Geometry check sheet. Reference: the model listing, model coordinates, mm. A direction names the side the tool comes from. Round coordinates to 2 decimals unless told otherwise and drop trailing zeros. Order: outer loops, then holes, each group sorted by start corner. A loop starts at its lowest first (then second) coordinate and runs counter-clockwise, first axis right, second up. Notation, with made-up numbers: M 26.25,47.5 L 48.25,47.5 A26 cw 48.25,86.5 Z; hole C 65.25,-21 d10. An arc over 180 degrees is marked long. Return JSON: item names as keys, results as strings. Group by question number.
```python
from build123d import *

# Parameters (mm, degrees)
SKETCH1_R           = 11.5
BOSS_EXTRUDE1_DEPTH = 5.3
BOSS_EXTRUDE2_START = 1
SKETCH2_R           = 11.5
BOSS_EXTRUDE2_DEPTH = 1
BOSS_EXTRUDE3_DEPTH = 6.3
FILLET1_R           = 5
CHAMFER1_SIZE       = 1
CUT_EXTRUDE1_REACH  = 32.016
SKETCH4_R           = 4.1


with BuildPart() as part:
    # Sketch1 → Boss-Extrude1 (new body)
    with BuildSketch(Plane.XY):
        Circle(SKETCH1_R)
        Polygon((0, 7.621023553), (-6.6, 3.810511777), (-6.6, -3.810511777), (0, -7.621023553), (6.6, -3.810511777), (6.6, 3.810511777), align=None, mode=Mode.SUBTRACT)
    extrude(amount=-BOSS_EXTRUDE1_DEPTH)

    # Sketch2 → Boss-Extrude2 (add)
    with BuildSketch(Plane.XY.offset(BOSS_EXTRUDE2_START)):
        Circle(SKETCH2_R)
    extrude(amount=-BOSS_EXTRUDE2_DEPTH)

    # Sketch3 → Boss-Extrude3 (add)
    with BuildSketch(Plane.XY.offset(1)):
        with BuildLine():
            Line((4, -23), (4, -10.781929326))
            ThreePointArc((4, -10.781929326), (0, -11.5), (-4, -10.781929326))
            Line((-4, -10.781929326), (-4, -23))
            ThreePointArc((-4, -23), (0, -27), (4, -23))
        make_face()
    extrude(amount=-BOSS_EXTRUDE3_DEPTH)

    # Fillet1
    fillet1_edges = [part.edges().sort_by_distance(p)[0] for p in [
        (4, -10.781929326, -2.15),
        (-4, -10.781929326, -2.15),
    ]]
    fillet(fillet1_edges, radius=FILLET1_R)

    # Chamfer1
    chamfer1_edges = [part.edges().sort_by_distance(p)[0] for p in [
        (0, -27, 1),
        (0, 11.5, 1),
        (-4, -18.414658343, 1),
        (4, -18.414658343, 1),
        (-4.604754635, -11.445660213, 1),
        (4.604754635, -11.445660213, 1),
    ]]
    chamfer(chamfer1_edges, length=CHAMFER1_SIZE)

    # Sketch4 → Cut-Extrude1 (cut, up to next)
    with BuildSketch(Plane.XY.offset(1), mode=Mode.PRIVATE) as cut_extrude1_sk1:
        Circle(SKETCH4_R)
    cut_extrude1_tool1 = extrude(cut_extrude1_sk1.sketch, amount=-CUT_EXTRUDE1_REACH, mode=Mode.PRIVATE) & part.part
    add(cut_extrude1_tool1.solids().sort_by_distance((0, 0, 1))[0], mode=Mode.SUBTRACT)


solid = part.part
```
Q1. Set-up check for faces 1 (the face through (-4, -18, -3)), 2 (the face through (-6.6, 0, -3)), 3 (the face through (3.5, -18.5, 0.5)): record each of +Z, -Z, +X, -X, +Y, -Y from which the full face is reachable in a straight line by a thin tool's end or side.
Q2. Material ranges on line 1 along X through (y, z) = (6.5, -4.75); line 2 along Y through (x, z) = (0, 0.7); line 3 along X through (y, z) = (-23, -4), recorded low to high.
Q3. Depth check by flat-ended pin: pin 1 Ø2.5 at (y, z) = (-1, -2) entering from -X; pin 2 Ø3 at (y, z) = (-2.5, -1) entering from +X. Enter the tip coordinate at first touch or a pass-through.
Q4. Section check B-B on z = -2.5. Record the cut outline in (x, y).
Q5. Section check D-D on z = 0.5. Record the cut outline in (x, y), plus the area to 3 significant figures.
Q6. Release check for a two-part mould opening along Y. For faces 4 (the face through (6.6, 0, -3)), 5 (the face through (4, -18, -3)), 6 (the face through (0, -27, -3)) record: +Y half, -Y half, draft (parallel to the pull), parting line (faces both ways), or undercut.
Q7. Section check A-A on y = 0. Record the cut outline in (x, z).
Q8. Section check C-C on y = -15.5. Record the cut outline in (x, z).
Geometry check:
{
 "1": {"face 1": "+Z, -Z, -X, -Y", "face 2": "-Z", "face 3": "+Z, +X, -Y"},
 "2": {"line 1": "x = -9.49 to -1.94, 1.94 to 9.49", "line 2": "y = -26.3 to -4.1, 4.1 to 10.8", "line 3": "x = -4 to 4"},
 "3": {"pin 1": "stops at x = -11.5", "pin 2": "stops at x = 11.46"},
 "4": {"outline": "M -6.27,-9.64 A5 cw -4,-13.83 L -4,-23 A4 ccw 4,-23 L 4,-13.83 A5 cw 6.27,-9.64 A11.5 ccw long Z; hole M -6.6,-3.81 L 0,-7.62 L 6.6,-3.81 L 6.6,3.81 L 0,7.62 L -6.6,3.81 Z"},
 "5": {"outline": "M -6,-9.22 A5.5 cw -3.5,-13.83 L -3.5,-23 A3.5 ccw 3.5,-23 L 3.5,-13.83 A5.5 cw 6,-9.22 A11 ccw long Z; hole C 0,0 d8.2", "area": "435 mm^2"},
 "6": {"face 4": "undercut", "face 5": "draft", "face 6": "-Y half"},
 "7": {"outline": "M -11.5,-5.3 L -6.6,-5.3 L -6.6,0 L -4.1,0 L -4.1,1 L -10.5,1 L -11.5,0 Z; M 4.1,0 L 6.6,0 L 6.6,-5.3 L 11.5,-5.3 L 11.5,0 L 10.5,1 L 4.1,1 Z"},
 "8": {"outline": "M -4,-5.3 L 4,-5.3 L 4,0 L 3,1 L -3,1 L -4,0 Z"}
}
